The model under review builds one solid part; all positions refer to its coordinate system, in mm. A direction names the side the tool comes from. Give positions to 0.01 mm unless a question says otherwise; leave off trailing zeros. Order: outer loops, then holes, each group sorted by start corner. A loop starts at its lowest first (then second) coordinate and runs counter-clockwise, first axis right, second up. Notation, with made-up numbers: (22, -24) - (49, -24) arc R10 cw to (49, -6) - close; hole circle Ø8 at (-39.75, 52.25). An arc over 180 degrees is marked (long way). Put each result on its own line as item: value.
```python
from build123d import *

# Parameters (mm, degrees)
SKETCH1_R           = 12.5
BOSS_EXTRUDE1_DEPTH = 4
SKETCH2_R           = 8.45
BOSS_EXTRUDE2_DEPTH = 5
SKETCH3_R           = 6.925
BOSS_EXTRUDE3_DEPTH = 2.3
SKETCH4_R           = 8.45
BOSS_EXTRUDE4_DEPTH = 11
SKETCH5_R           = 5.45
BOSS_EXTRUDE5_DEPTH = 3.2
SKETCH6_R           = 5.45
BOSS_EXTRUDE7_DEPTH = 5
SKETCH7_R           = 3.5
CUT_EXTRUDE1_DEPTH  = 36.252659474
CHAMFER1_START      = 25.5
CHAMFER1_2_DEPTH    = 5.5
FILLET1_R           = 0.5


with BuildPart() as part:
    # Sketch1 → Boss-Extrude1 (new body)
    with BuildSketch(Plane(origin=(0, 0, 0), x_dir=(1, 0, 0), z_dir=(0, 1, 0))):
        with Locations(Location((0, 0, 0), (0, 0, 270))):
            Circle(SKETCH1_R)
    extrude(amount=BOSS_EXTRUDE1_DEPTH)

    # Sketch2 → Boss-Extrude2 (add)
    with BuildSketch(Plane(origin=(0, 4, 0), x_dir=(1, 0, 0), z_dir=(0, 1, 0))):
        with Locations(Location((0, 0, 0), (0, 0, 270))):
            Circle(SKETCH2_R)
    extrude(amount=BOSS_EXTRUDE2_DEPTH)

    # Sketch3 → Boss-Extrude3 (add)
    with BuildSketch(Plane(origin=(0, 9, 0), x_dir=(1, 0, 0), z_dir=(0, 1, 0))):
        with Locations(Location((0, 0, 0), (0, 0, 270))):
            Circle(SKETCH3_R)
    extrude(amount=BOSS_EXTRUDE3_DEPTH)

    # Sketch4 → Boss-Extrude4 (add)
    with BuildSketch(Plane(origin=(0, 11.3, 0), x_dir=(1, 0, 0), z_dir=(0, 1, 0))):
        with Locations(Location((0, 0, 0), (0, 0, 270))):
            Circle(SKETCH4_R)
    extrude(amount=BOSS_EXTRUDE4_DEPTH)

    # Sketch5 → Boss-Extrude5 (add)
    with BuildSketch(Plane(origin=(0, 22.3, 0), x_dir=(1, 0, 0), z_dir=(0, 1, 0))):
        with Locations(Location((0, 0, 0), (0, 0, 270))):
            Circle(SKETCH5_R)
    extrude(amount=BOSS_EXTRUDE5_DEPTH)

    # Sketch6 → Boss-Extrude7 (add)
    with BuildSketch(Plane(origin=(0, 25.5, 0), x_dir=(1, 0, 0), z_dir=(0, 1, 0))):
        with Locations(Location((0, 0, 0), (0, 0, 270))):
            Circle(SKETCH6_R)
        with BuildLine():
            Line((-8.45, 0), (-5.45, 0))
            ThreePointArc((-5.45, 0), (-5.035143452, 2.085624706), (-3.853731957, 3.853731957))
            Line((-3.853731957, 3.853731957), (-5.975052301, 5.975052301))
            ThreePointArc((-5.975052301, 5.975052301), (-7.80678205, 3.233675003), (-8.45, 0))
        make_face()
        with BuildLine():
            ThreePointArc((0, -5.45), (-2.085624706, -5.035143452), (-3.853731957, -3.853731957))
            Line((-3.853731957, -3.853731957), (-5.975052301, -5.975052301))
            ThreePointArc((-5.975052301, -5.975052301), (-3.233675003, -7.80678205), (0, -8.45))
            Line((0, -8.45), (0, -5.45))
        make_face()
        with BuildLine():
            ThreePointArc((5.45, 0), (5.035143452, -2.085624706), (3.853731957, -3.853731957))
            Line((3.853731957, -3.853731957), (5.975052301, -5.975052301))
            ThreePointArc((5.975052301, -5.975052301), (7.80678205, -3.233675003), (8.45, 0))
            Line((8.45, 0), (5.45, 0))
        make_face()
        with BuildLine():
            Line((0, 8.45), (0, 5.45))
            ThreePointArc((0, 5.45), (2.085624706, 5.035143452), (3.853731957, 3.853731957))
            Line((3.853731957, 3.853731957), (5.975052301, 5.975052301))
            ThreePointArc((5.975052301, 5.975052301), (3.233675003, 7.80678205), (0, 8.45))
        make_face()
    extrude(amount=BOSS_EXTRUDE7_DEPTH)

    # Sketch7 → Cut-Extrude1 (cut, through all)
    with BuildSketch(Plane(origin=(0, 30.5, 0), x_dir=(1, 0, 0), z_dir=(0, 1, 0))):
        with Locations(Location((0, 0, 0), (0, 0, 270))):
            Circle(SKETCH7_R)
    extrude(amount=-CUT_EXTRUDE1_DEPTH, mode=Mode.SUBTRACT)

    # Chamfer1: read off the stored shape, not the designer's step
    # Chamfer1 outline → Chamfer1 (revolve, cut)
    with BuildSketch(Plane.XY):
        Polygon((12.5, 0.5), (12, 0), (12.5, 0), align=None)
        Polygon((12, 4), (12.5, 3.5), (12.5, 4), align=None)
        Polygon((7.95, 9), (8.45, 8.5), (8.45, 9), align=None)
        Polygon((7.95, 11.3), (8.45, 11.3), (8.45, 11.8), align=None)
        Polygon((7.95, 22.3), (8.45, 21.8), (8.45, 22.3), align=None)
        Polygon((7.95, 30.5), (8.45, 30), (8.45, 30.5), align=None)
        Polygon((3.5, 30), (4, 30.5), (3.5, 30.5), align=None)
    revolve(axis=Axis((0, 0, 0), (0, 1, 0)), mode=Mode.SUBTRACT)

    # Chamfer1 2 outline → Chamfer1 2 (cut)
    with BuildSketch(Plane(origin=(0, 0, 0), x_dir=(1, 0, 0), z_dir=(0, 1, 0)).offset(CHAMFER1_START)):
        with BuildLine():
            Line((8.45, 0), (7.93426115, 0))
            Line((7.93426115, 0), (8.433271285, -0.531446541))
            ThreePointArc((8.433271285, -0.531446541), (8.445816786, -0.265854883), (8.45, 0))
        make_face()
        with BuildLine():
            ThreePointArc((5.975052301, -5.975052301), (6.160082112, -5.784106531), (6.339012766, -5.587433861))
            Line((6.339012766, -5.587433861), (5.610369863, -5.610369863))
            Line((5.610369863, -5.610369863), (5.975052301, -5.975052301))
        make_face()
        with BuildLine():
            ThreePointArc((5.975052301, 5.975052301), (5.784106531, 6.160082112), (5.587433861, 6.339012766))
            Line((5.587433861, 6.339012766), (5.610369863, 5.610369863))
            Line((5.610369863, 5.610369863), (5.975052301, 5.975052301))
        make_face()
        with BuildLine():
            Line((0, 7.93426115), (0.531446541, 8.433271285))
            ThreePointArc((0.531446541, 8.433271285), (0.265854883, 8.445816786), (0, 8.45))
            Line((0, 8.45), (0, 7.93426115))
        make_face()
        with BuildLine():
            ThreePointArc((-5.975052301, -5.975052301), (-5.784106531, -6.160082112), (-5.587433861, -6.339012766))
            Line((-5.587433861, -6.339012766), (-5.610369863, -5.610369863))
            Line((-5.610369863, -5.610369863), (-5.975052301, -5.975052301))
        make_face()
        with BuildLine():
            Line((0, -7.93426115), (-0.531446541, -8.433271285))
            ThreePointArc((-0.531446541, -8.433271285), (-0.265854883, -8.445816786), (0, -8.45))
            Line((0, -8.45), (0, -7.93426115))
        make_face()
        with BuildLine():
            ThreePointArc((-5.975052301, 5.975052301), (-6.160082112, 5.784106531), (-6.339012766, 5.587433861))
            Line((-6.339012766, 5.587433861), (-5.610369863, 5.610369863))
            Line((-5.610369863, 5.610369863), (-5.975052301, 5.975052301))
        make_face()
        with BuildLine():
            Line((-7.93426115, 0), (-8.433271285, 0.531446541))
            ThreePointArc((-8.433271285, 0.531446541), (-8.445816786, 0.265854883), (-8.45, 0))
            Line((-8.45, 0), (-7.93426115, 0))
        make_face()
    extrude(amount=CHAMFER1_2_DEPTH, mode=Mode.SUBTRACT)

    # Chamfer1 3 outline → Chamfer1 3 (revolve, cut)
    with BuildSketch(Plane.XY):
        Polygon((8.45, 26), (7.95, 25.5), (8.45, 25.5), align=None)
    revolve(axis=Axis((0, 0, 0), (0, 1, 0)), mode=Mode.SUBTRACT)

    # Fillet1
    fillet1_edges = [part.edges().sort_by_distance(p)[0] for p in [
        (0, 11.3, -6.925),
        (0, 9, -6.925),
    ]]
    fillet(fillet1_edges, radius=FILLET1_R)


solid = part.part
```
(1) Clearance check with flat-ended pins moving along their axes: pin 1 Ø4 at (y, z) = (7.5, 6.5) entering from -X; pin 2 Ø12 at (x, y) = (-4.5, 14) entering from +Z; pin 3 Ø3 at (y, z) = (8, -9) entering from -X; pin 4 Ø4 at (x, z) = (0, 0) entering from +Y. State where each tip first meets the part, or that it passes through.
The answers:
pin 1: x = -7.15
pin 2: z = 8.45
pin 3: x = -3.89
pin 4: through
(2) For faces 1 (the flat face through (5, 28, -5)), 2 (the cylindrical face through (3.27, 27.97, -7.79)), 3 (the cylindrical face through (7.79, 27.97, 3.27)), list the 3-axis set-ups (+Z, -Z, +X, -X, +Y, -Y) from which the entire face can be reached by the end or side of a thin tool; tool diameter is ignored.
The answers:
face 1: +X, +Y
face 2: -Z, +X, +Y
face 3: +Z, +X, +Y
(3) Take a section at A-A, the plane y = 15.5. Write out the cut boundary in (x, z).
The answers:
outline: circle Ø16.9 at (0, 0); hole circle Ø7 at (0, 0)
(4) The part is to be moulded in two halves that separate along Y. For faces 4 (the cylindrical face through (2.54, 16.73, 8.06)), 5 (the flat face through (-1.7, 22.3, -5.4)), 6 (the conical face through (7.453, 25.635, 3.135)), 7 (the conical face through (3.138, 30.358, -7.459)), say which applies: pulls with the +Y half, pulls with the -Y half, needs draft (parallel to the pull), parting line crosses it, or undercut.
The answers:
face 4: needs draft
face 5: undercut
face 6: undercut
face 7: pulls with the +Y half
(5) Wall thickness on L1, parallel to Z at x = 0, y = 23; L2, parallel to Y at x = 1, z = -8; L3, parallel to X at y = 16.75, z = 0: over which ranges is each line inside the solid? List them lowest first.
The answers:
L1: -5.45 to -3.5, 3.5 to 5.45
L2: 0 to 8.89, 11.41 to 22.19, 25.61 to 30.39
L3: -8.45 to -3.5, 3.5 to 8.45
